from build123d import *

# Parameters (mm, degrees)
F0_W     = 12
F0_H     = 12
F1_DEPTH = 6


with BuildPart() as f1:
    # F0 (on Top) → F1 (new body)
    with BuildSketch(Plane.XY):
        with BuildLine():
            ThreePointArc((18.0019915499, 4.8236190979), (18.6486934227, 5.0431448029), (19.3185165258, 5.1763809021))
            ThreePointArc((19.3185165258, 5.1763809021), (17.3205080757, 10), (14.1421356237, 14.1421356237))
            ThreePointArc((14.1421356237, 14.1421356237), (13.6918382257, 13.62866985), (13.178372452, 13.178372452))
            ThreePointArc((13.178372452, 13.178372452), (12.7989481428, 7.3894761556), (18.0019915499, 4.8236190979))
        make_face()
        with BuildLine():
            ThreePointArc((14.1421356237, 14.1421356237), (17.3205080757, 10), (19.3185165258, 5.1763809021))
            ThreePointArc((19.3185165258, 5.1763809021), (21.6616505733, 7.0993413189), (22.5415557645, 10))
            ThreePointArc((22.5415557645, 10), (19.6297184195, 14.6826153543), (14.1421356237, 14.1421356237))
        make_face()
        with BuildLine():
            ThreePointArc((22.5415557645, -10), (21.6616505733, -7.0993413189), (19.3185165258, -5.1763809021))
            ThreePointArc((19.3185165258, -5.1763809021), (17.3205080757, -10), (14.1421356237, -14.1421356237))
            ThreePointArc((14.1421356237, -14.1421356237), (19.6297184195, -14.6826153543), (22.5415557645, -10))
        make_face()
        with BuildLine():
            ThreePointArc((14.1421356237, -14.1421356237), (17.3205080757, -10), (19.3185165258, -5.1763809021))
            ThreePointArc((19.3185165258, -5.1763809021), (18.6486934227, -5.0431448029), (18.0019915499, -4.8236190979))
            ThreePointArc((18.0019915499, -4.8236190979), (12.7989481428, -7.3894761556), (13.178372452, -13.178372452))
            ThreePointArc((13.178372452, -13.178372452), (13.6918382257, -13.62866985), (14.1421356237, -14.1421356237))
        make_face()
        with BuildLine():
            ThreePointArc((18.0019915499, -4.8236190979), (14.7789523112, 0), (18.0019915499, 4.8236190979))
            ThreePointArc((18.0019915499, 4.8236190979), (12.7989481428, 7.3894761556), (13.178372452, 13.178372452))
            ThreePointArc((13.178372452, 13.178372452), (7.3894761556, 12.7989481428), (4.8236190979, 18.0019915499))
            ThreePointArc((4.8236190979, 18.0019915499), (0, 14.7789523112), (-4.8236190979, 18.0019915499))
            ThreePointArc((-4.8236190979, 18.0019915499), (-4.7901309751, 17.6619809324), (-4.7789523112, 17.3205080757))
            ThreePointArc((-4.7789523112, 17.3205080757), (-7.6907896561, 12.6378927214), (-13.178372452, 13.178372452))
            ThreePointArc((-13.178372452, 13.178372452), (-12.3765407116, 11.6782507774), (-12.0994603869, 10))
            ThreePointArc((-12.0994603869, 10), (-13.8780321316, 6.0746085108), (-18.0019915499, 4.8236190979))
            ThreePointArc((-18.0019915499, 4.8236190979), (-15.6588575024, 2.9006586811), (-14.7789523112, 0))
            ThreePointArc((-14.7789523112, 0), (-15.6588575024, -2.9006586811), (-18.0019915499, -4.8236190979))
            ThreePointArc((-18.0019915499, -4.8236190979), (-13.8780321316, -6.0746085108), (-12.0994603869, -10))
            ThreePointArc((-12.0994603869, -10), (-12.3765407116, -11.6782507774), (-13.178372452, -13.178372452))
            ThreePointArc((-13.178372452, -13.178372452), (-7.6907896561, -12.6378927214), (-4.7789523112, -17.3205080757))
            ThreePointArc((-4.7789523112, -17.3205080757), (-4.7901309751, -17.6619809324), (-4.8236190979, -18.0019915499))
            ThreePointArc((-4.8236190979, -18.0019915499), (0, -14.7789523112), (4.8236190979, -18.0019915499))
            ThreePointArc((4.8236190979, -18.0019915499), (7.3894761556, -12.7989481428), (13.178372452, -13.178372452))
            ThreePointArc((13.178372452, -13.178372452), (12.7989481428, -7.3894761556), (18.0019915499, -4.8236190979))
        make_face()
        Rectangle(F0_W, F0_H, mode=Mode.SUBTRACT)
        with BuildLine():
            ThreePointArc((4.8236190979, 18.0019915499), (4.9568551971, 18.6718146529), (5.1763809021, 19.3185165258))
            ThreePointArc((5.1763809021, 19.3185165258), (0, 20), (-5.1763809021, 19.3185165258))
            ThreePointArc((-5.1763809021, 19.3185165258), (-4.9568551971, 18.6718146529), (-4.8236190979, 18.0019915499))
            ThreePointArc((-4.8236190979, 18.0019915499), (0, 14.7789523112), (4.8236190979, 18.0019915499))
        make_face()
        with BuildLine():
            ThreePointArc((-5.1763809021, 19.3185165258), (0, 20), (5.1763809021, 19.3185165258))
            ThreePointArc((5.1763809021, 19.3185165258), (5.2098690249, 19.6585271433), (5.2210476888, 20))
            ThreePointArc((5.2210476888, 20), (-0.3414728567, 25.2098690249), (-5.1763809021, 19.3185165258))
        make_face()
        with BuildLine():
            ThreePointArc((5.2210476888, -20), (5.2098690249, -19.6585271433), (5.1763809021, -19.3185165258))
            ThreePointArc((5.1763809021, -19.3185165258), (0, -20), (-5.1763809021, -19.3185165258))
            ThreePointArc((-5.1763809021, -19.3185165258), (-0.3414728567, -25.2098690249), (5.2210476888, -20))
        make_face()
        with BuildLine():
            ThreePointArc((-5.1763809021, -19.3185165258), (0, -20), (5.1763809021, -19.3185165258))
            ThreePointArc((5.1763809021, -19.3185165258), (4.9568551971, -18.6718146529), (4.8236190979, -18.0019915499))
            ThreePointArc((4.8236190979, -18.0019915499), (0, -14.7789523112), (-4.8236190979, -18.0019915499))
            ThreePointArc((-4.8236190979, -18.0019915499), (-4.9568551971, -18.6718146529), (-5.1763809021, -19.3185165258))
        make_face()
        with BuildLine():
            ThreePointArc((-13.178372452, 13.178372452), (-13.6918382257, 13.62866985), (-14.1421356237, 14.1421356237))
            ThreePointArc((-14.1421356237, 14.1421356237), (-17.3205080757, 10), (-19.3185165258, 5.1763809021))
            ThreePointArc((-19.3185165258, 5.1763809021), (-18.6486934227, 5.0431448029), (-18.0019915499, 4.8236190979))
            ThreePointArc((-18.0019915499, 4.8236190979), (-13.8780321316, 6.0746085108), (-12.0994603869, 10))
            ThreePointArc((-12.0994603869, 10), (-12.3765407116, 11.6782507774), (-13.178372452, 13.178372452))
        make_face()
        with BuildLine():
            ThreePointArc((-19.3185165258, 5.1763809021), (-17.3205080757, 10), (-14.1421356237, 14.1421356237))
            ThreePointArc((-14.1421356237, 14.1421356237), (-21.8420680086, 12.6105238444), (-19.3185165258, 5.1763809021))
        make_face()
        with BuildLine():
            ThreePointArc((-19.3185165258, -5.1763809021), (-21.8420680086, -12.6105238444), (-14.1421356237, -14.1421356237))
            ThreePointArc((-14.1421356237, -14.1421356237), (-17.3205080757, -10), (-19.3185165258, -5.1763809021))
        make_face()
        with BuildLine():
            ThreePointArc((-19.3185165258, -5.1763809021), (-17.3205080757, -10), (-14.1421356237, -14.1421356237))
            ThreePointArc((-14.1421356237, -14.1421356237), (-13.6918382257, -13.62866985), (-13.178372452, -13.178372452))
            ThreePointArc((-13.178372452, -13.178372452), (-12.3765407116, -11.6782507774), (-12.0994603869, -10))
            ThreePointArc((-12.0994603869, -10), (-13.8780321316, -6.0746085108), (-18.0019915499, -4.8236190979))
            ThreePointArc((-18.0019915499, -4.8236190979), (-18.6486934227, -5.0431448029), (-19.3185165258, -5.1763809021))
        make_face()
    extrude(amount=F1_DEPTH)


solid = f1.part
Read the model definition and answer for the solid it produces. Units are mm, in the model's axes. A direction names the side the tool comes from. Round coordinates to 2 decimals unless told otherwise and drop trailing zeros. Loops run counter-clockwise (first coordinate to the right, second up) from the corner with the lowest first, then second, coordinate; pieces in that order, holes last.
Q1. Consider probe 1 along X at (y, z) = (-14, 4.95); probe 2 along X at (y, z) = (0, 2.5); probe 3 along Y at (x, z) = (16.5, 0.3). Determine where each line is inside the solid, lowest interval first.
Q2. Each of these flat-tipped pins is pushed along its axis until it touches: pin 1 (3 mm diameter, centred on x = 3, z = 4.5, fed in from +Y); pin 2 (1 mm diameter, centred on x = 9, z = 3.5, fed in from +Y); pin 3 (3 mm diameter, centred on y = 16, z = 5, fed in from -X). Where does it stop, or does it pass through?
Q3. Determine the mould class of faces 1 (the face through (-6, 0, 3)), 2 (the face through (10, 0, 0)) for opening direction Y: released by +Y, released by -Y, zero draft, split by the parting line, or undercut.
Q4. Section B-B on y = -3.5 is taken. Write down the section's boundary in (x, z).
Q5. Section C-C on x = 12.5 is taken. Write down the section's boundary in (y, z).
Q6. Which of the six approach directions +Z, -Z, +X, -X, +Y, -Y give full straight-line access (tool end or side, diameter ignored) to faces 3 (the face through (10, 0, 6)), 4 (the face through (0, -6, 3))?
Q7. Section D-D on x = -9 is taken. Write down the section's boundary in (y, z).
Q8. Section A-A on x = 0 is taken. Write down the section's boundary in (y, z).
Output:
1. probe 1: x = -20.68 to -14.03, -5.97 to 5.97, 14.03 to 20.68
1. probe 2: x = -14.78 to -6, 6 to 14.78
1. probe 3: y = -15.16 to -3.87, 3.87 to 15.16
2. pin 1: stops at y = 25
2. pin 2: stops at y = 12.32
2. pin 3: stops at x = -19.97
3. face 1: undercut
3. face 2: zero draft
4. outline: (-16.13, 0) - (-6, 0) - (-6, 6) - (-16.13, 6) - close; (6, 0) - (16.13, 0) - (16.13, 6) - (6, 6) - close
5. outline: (-12.74, 0) - (12.74, 0) - (12.74, 6) - (-12.74, 6) - close
6. face 3: +Z, +X, -X, +Y, -Y
6. face 4: +Z, -Z
7. outline: (-12.2, 0) - (12.2, 0) - (12.2, 6) - (-12.2, 6) - close
8. outline: (-25.22, 0) - (-6, 0) - (-6, 6) - (-25.22, 6) - close; (6, 0) - (25.22, 0) - (25.22, 6) - (6, 6) - close
